Verification items for the finished model (mm, model axes). Round coordinates to 2 decimals unless told otherwise and drop trailing zeros. Loops run counter-clockwise (first coordinate to the right, second up) from the corner with the lowest first, then second, coordinate; pieces in that order, holes last. Notation, with made-up numbers: M 76,72.5 L 107,72.5 A18 ccw 107,77.5 Z; hole C -31,68.25 d1. An arc over 180 degrees is marked long. Answer as CSV lines item,"result".
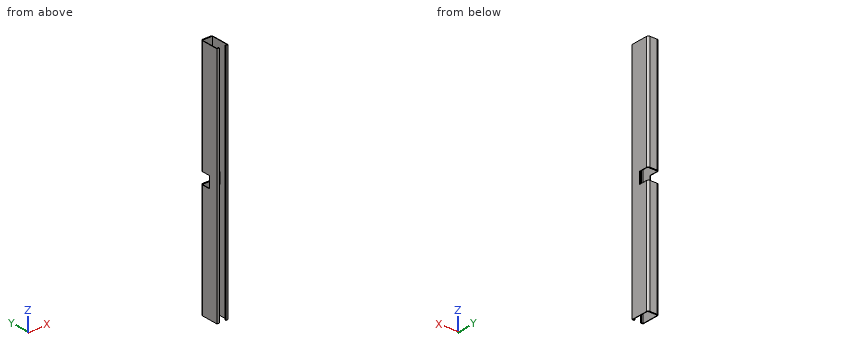
```python
from build123d import *

# Parameters (mm, degrees)
BOSS_EXTRUDE1_DEPTH            = 250
CUT_EXTRUDE1_REACH             = 255.441
SKETCH2_W                      = 24
SKETCH2_H                      = 21.42
CUT_EXTRUDE1_DIRECTION_2_REACH = 255.441


with BuildPart() as part:
    # Sketch1 → Boss-Extrude1 (new, symmetric)
    with BuildSketch(Plane.XY):
        with BuildLine():
            Line((6.785, 0), (6.785, 1.73))
            Line((6.785, 1.73), (10.485, 1.73))
            Line((10.485, 1.73), (10.485, 37.58))
            Line((10.485, 37.58), (-10.485, 37.58))
            Line((-10.485, 37.58), (-10.485, 1.73))
            Line((-10.485, 1.73), (-6.785, 1.73))
            Line((-6.785, 1.73), (-6.785, 0))
            Line((-6.785, 0), (-11.5, 0))
            Line((-11.5, 0), (-11.5, 36))
            ThreePointArc((-11.5, 36), (-10.328427125, 38.828427125), (-7.5, 40))
            Line((-7.5, 40), (7.5, 40))
            ThreePointArc((7.5, 40), (10.328427125, 38.828427125), (11.5, 36))
            Line((11.5, 36), (11.5, 0))
            Line((11.5, 0), (6.785, 0))
        make_face()
    extrude(amount=BOSS_EXTRUDE1_DEPTH, both=True)

    # Sketch2 → Cut-Extrude1 (cut, up to next)
    with BuildSketch(Plane(origin=(0, 0, 0), x_dir=(0, 0, -1), z_dir=(1, 0, 0)), mode=Mode.PRIVATE) as cut_extrude1_sk1:
        with Locations((0, 29.29)):
            Rectangle(SKETCH2_W, SKETCH2_H)
    cut_extrude1_tool1 = extrude(cut_extrude1_sk1.sketch, amount=-CUT_EXTRUDE1_REACH, mode=Mode.PRIVATE) & part.part
    add(cut_extrude1_tool1.solids().sort_by_distance((0, 29.29, 0))[0], mode=Mode.SUBTRACT)

    # Sketch2 → Cut-Extrude1 direction 2 (cut, up to next)
    with BuildSketch(Plane(origin=(0, 0, 0), x_dir=(0, 0, -1), z_dir=(1, 0, 0)), mode=Mode.PRIVATE) as cut_extrude1_direction_2_sk1:
        with Locations((0, 29.29)):
            Rectangle(SKETCH2_W, SKETCH2_H)
    cut_extrude1_direction_2_tool1 = extrude(cut_extrude1_direction_2_sk1.sketch, amount=CUT_EXTRUDE1_DIRECTION_2_REACH, mode=Mode.PRIVATE) & part.part
    add(cut_extrude1_direction_2_tool1.solids().sort_by_distance((0, 29.29, 0))[0], mode=Mode.SUBTRACT)


solid = part.part
```
1) Go/stop test with flat-tipped pins: pin 1 (0.5 mm diameter, centred on x = -11, z = -5.5, fed in from +Y); pin 2 (1.1 mm diameter, centred on x = -9.5, z = -111, fed in from +Y). Record where each tip stops, or that it passes through.
Here are the results:
pin 1,"stops at y = 18.58"
pin 2,"stops at y = 39.73"
2) Material ranges on probe 1 along X at (y, z) = (31, -225.5) (3 decimals); probe 2 along Y at (x, z) = (-7.5, 45); probe 3 along Y at (x, z) = (8.75, -106), recorded low to high.
Here are the results:
probe 1,"x = -11.5 to -10.485, 10.485 to 11.5"
probe 2,"y = 0 to 1.73, 37.58 to 40"
probe 3,"y = 0 to 1.73, 37.58 to 39.8"
3) Section check A-A (x = 1.25). Record the cut outline in (y, z), plus the area to 3 significant figures.
Here are the results:
outline,"M 37.58,-250 L 40,-250 L 40,-12 L 37.58,-12 Z; M 37.58,12 L 40,12 L 40,250 L 37.58,250 Z"
area,"1,150 mm^2"
4) Section check C-C (z = 220.5). Record the cut outline in (x, y) (3 decimals), plus the area to 3 significant figures.
Here are the results:
outline,"M -11.5,0 L -6.785,0 L -6.785,1.73 L -10.485,1.73 L -10.485,37.58 L 10.485,37.58 L 10.485,1.73 L 6.785,1.73 L 6.785,0 L 11.5,0 L 11.5,36 A4 ccw 7.5,40 L -7.5,40 A4 ccw -11.5,36 Z"
area,"138 mm^2"
5) Section check B-B (y = 25.5). Record the cut outline in (x, z) (3 decimals).
Here are the results:
outline,"M -11.5,-250 L -10.485,-250 L -10.485,-12 L -11.5,-12 Z; M -11.5,12 L -10.485,12 L -10.485,250 L -11.5,250 Z; M 10.485,-250 L 11.5,-250 L 11.5,-12 L 10.485,-12 Z; M 10.485,12 L 11.5,12 L 11.5,250 L 10.485,250 Z"
